from build123d import *

# Parameters (mm, degrees)
SKETCH1_R           = 7.14375
BOSS_EXTRUDE1_DEPTH = 3.175


with BuildPart() as part:
    # Sketch1 → Boss-Extrude1 (new, symmetric)
    with BuildSketch(Plane.XY):
        Polygon((0, 88.9), (0, 0), (88.9, 0), (88.9, 41.275), (41.275, 41.275), (41.275, 88.9), align=None)
        with Locations((20.6375, 20.6375)):
            Circle(SKETCH1_R, mode=Mode.SUBTRACT)
        with Locations((20.6375, 68.2625)):
            Circle(SKETCH1_R, mode=Mode.SUBTRACT)
        with Locations((68.2625, 20.6375)):
            Circle(SKETCH1_R, mode=Mode.SUBTRACT)
    extrude(amount=BOSS_EXTRUDE1_DEPTH, both=True)


solid = part.part
The listing builds one solid part. Answer for the finished solid, in the listing's coordinates (mm). A direction names the side the tool comes from. Round coordinates to 2 decimals unless told otherwise and drop trailing zeros. Write each loop counter-clockwise with the first axis right and the second up, starting at its lowest first coordinate (ties: lowest second). Pieces come first, ordered by that corner, then holes. Notation, with made-up numbers: (0.25, 56.25) - (6.25, 56.25) arc R22 cw to (6.25, 84.25) - close; hole circle Ø11 at (-21, 32). An arc over 180 degrees is marked (long way). Use a Markdown table: item, result. Add a question column.
1. The part is cut by section C-C (x = 71.5). Write down the section's boundary in (y, z) (3 decimals), and give its area (3 significant figures).
2. The part is cut by section B-B (y = 66). Write down the section's boundary in (x, z) (1 decimal), and give its area (3 significant figures).
3. Flat-ended cylindrical pins translate along their axes: P1, Ø13, axis at x = 20.64, y = 20.64, coming from the +Z side; P2, Ø1.9, axis at x = 67.5, z = -0.5, coming from the +Y side (3 decimals). Find the tip coordinate at first contact, or state that the pin passes through.
4. The part is cut by section A-A (y = 22.5). Write down the section's boundary in (x, z) (3 decimals).
5. For a pull along Y with two mould halves and no side action, classify faces 3 (the face through (21, 88.9, 0)), 4 (the face through (0, 45, 0)), 5 (the face through (23.934, 61.925, -0.044)) as +Y half, -Y half, draft (parallel to the pull), parting line (faces both ways), or undercut.
6. The part is cut by section D-D (z = -0.25). Write down the section's boundary in (x, y) (1 decimal), and give its area (3 significant figures).
7. A tool of negligible diameter and unlimited length cuts with its end or side. For faces 1 (the face through (41.275, 65, 0)), 2 (the face through (88.9, 20, 0)), from which of +Z, -Z, +X, -X, +Y, -Y can it reach the whole face along a straight path? Write none if from no direction.
8. Consider line 1 (X direction, y = 68, z = 2.5) (3 decimals); line 2 (Y direction, x = 61, z = 0.5) (3 decimals); line 3 (X direction, y = 63, z = -0.25) (3 decimals). Determine where each line is inside the solid, lowest interval first.
Reported:
| question | item | result |
|---|---|---|
| 1 | outline | (0, -3.175) - (14.269, -3.175) - (14.269, 3.175) - (0, 3.175) - close; (27.006, -3.175) - (41.275, -3.175) - (41.275, 3.175) - (27.006, 3.175) - close |
| 1 | area | 181 mm^2 |
| 2 | outline | (0, -3.2) - (13.9, -3.2) - (13.9, 3.2) - (0, 3.2) - close; (27.4, -3.2) - (41.3, -3.2) - (41.3, 3.2) - (27.4, 3.2) - close |
| 2 | area | 176 mm^2 |
| 3 | P1 | through |
| 3 | P2 | y = 41.275 |
| 4 | outline | (0, -3.175) - (13.741, -3.175) - (13.741, 3.175) - (0, 3.175) - close; (27.534, -3.175) - (61.366, -3.175) - (61.366, 3.175) - (27.534, 3.175) - close; (75.159, -3.175) - (88.9, -3.175) - (88.9, 3.175) - (75.159, 3.175) - close |
| 5 | face 3 | +Y half |
| 5 | face 4 | draft |
| 5 | face 5 | undercut |
| 6 | outline | (0, 0) - (88.9, 0) - (88.9, 41.3) - (41.3, 41.3) - (41.3, 88.9) - (0, 88.9) - close; hole circle Ø14.3 at (20.6, 20.6); hole circle Ø14.3 at (20.6, 68.3); hole circle Ø14.3 at (68.3, 20.6) |
| 6 | area | 5,150 mm^2 |
| 7 | face 1 | +Z, -Z, +X, +Y |
| 7 | face 2 | +Z, -Z, +X, +Y, -Y |
| 8 | line 1 | 0 to 13.499, 27.776 to 41.275 |
| 8 | line 2 | 0 to 41.275 |
| 8 | line 3 | 0 to 15.806, 25.469 to 41.275 |
